Geometry: final body of the model. Coordinates: model frame, mm. Coordinates: 2 decimals unless noted, no trailing zeros. Write each loop counter-clockwise with the first axis right and the second up, starting at its lowest first coordinate (ties: lowest second). Pieces come first, ordered by that corner, then holes.
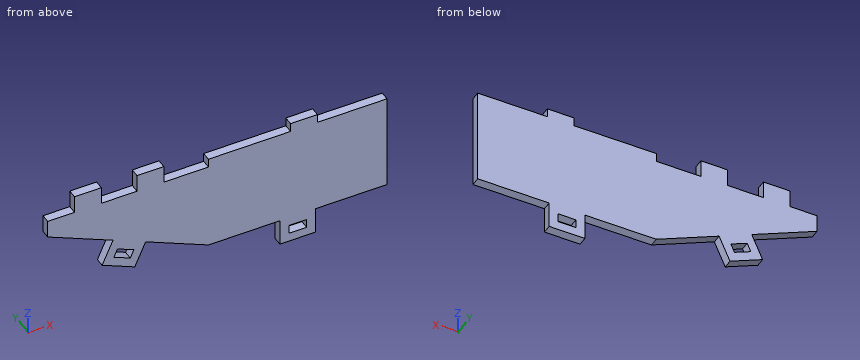
from build123d import *

# Parameters (mm, degrees)
SKETCH1_W           = 10
SKETCH1_H           = 5
BOSS_EXTRUDE1_DEPTH = 5


with BuildPart() as part:
    # Sketch1 → Boss-Extrude1 (new body)
    with BuildSketch(Plane(origin=(0, 0, 0), x_dir=(1, 0, 0), z_dir=(0, 1, 0))):
        Polygon((0, 0), (15, 0), (15, -10), (30, -10), (30, 0), (50, 0), (50, -10), (65, -10), (65, 0), (90, 0), (90, -5), (136, -5), (136, -10), (151, -10), (151, -5), (190, -5), (190, 50), (150, 50), (150, 65), (130, 65), (130, 50), (90, 50), (54.828692917, 34.368307963), (48.736615926, 48.075481193), (30.460384954, 39.952711871), (36.552461945, 26.245538642), (0, 10), align=None)
        Polygon((39.061482867, 32.832359245), (37.060135027, 37.414346459), (46.224109455, 41.417042137), (48.254801785, 36.847984394), align=None, mode=Mode.SUBTRACT)
        with Locations((140, 57.5)):
            Rectangle(SKETCH1_W, SKETCH1_H, mode=Mode.SUBTRACT)
    extrude(amount=BOSS_EXTRUDE1_DEPTH)


solid = part.part
Item 1: Material intervals for probe 1 along X at (y, z) = (4.05, 3); probe 2 along X at (y, z) = (2.6, 7); probe 3 along Z at (x, y) = (120, 2.1), sorted ascending.
Derived:
probe 1: x = 15 to 30, 50 to 65, 90 to 190
probe 2: x = 15 to 30, 50 to 65, 136 to 151
probe 3: z = -50 to 5
Item 2: Section A-A, the plane y = 1.9. State how many separate pieces and enclosed holes the cut face has, plus the area to 3 significant figures.
Derived:
separate pieces: 1
enclosed holes: 2
area: 9,070 mm2
Item 3: Section C-C, the plane x = 166.5. Output: boundary loops of the cut face in (y, z), plus the area to 3 significant figures.
Derived:
outline: (0, -50) - (5, -50) - (5, 5) - (0, 5) - close
area: 275 mm2
Item 4: Section B-B, the plane z = -22. Output: boundary loops of the cut face in (x, y), plus the area to 3 significant figures.
Derived:
outline: (27, 0) - (190, 0) - (190, 5) - (27, 5) - close
area: 815 mm2
Item 5: Pin query (flat end, axial travel): pin 1 (1 mm diameter, centred on y = 2, z = -53, fed in from +X); pin 2 (2.5 mm diameter, centred on x = 40.5, y = 2.5, fed in from +Z); pin 3 (2 mm diameter, centred on y = 3, z = -28, fed in from -X). Return the tip coordinate at first contact, or that it passes through.
Derived:
pin 1: stops at x = 150
pin 2: stops at z = 0
pin 3: stops at x = 35.33
